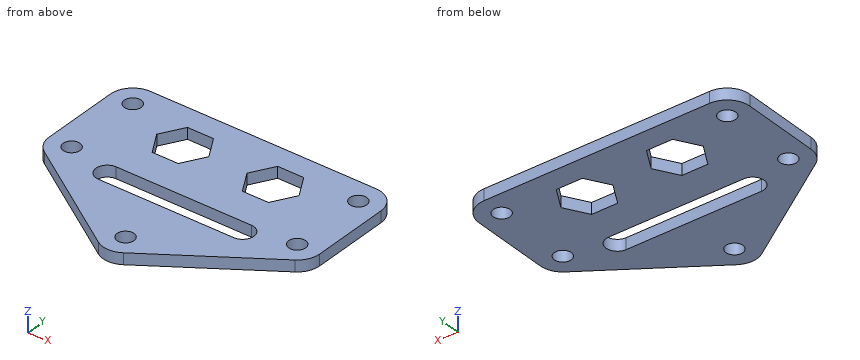
```python
from build123d import *

# Parameters (mm, degrees)
SKETCH1_R           = 4.7625
BOSS_EXTRUDE1_DEPTH = 6.35


with BuildPart() as part:
    # Sketch1 → Boss-Extrude1 (new body)
    with BuildSketch(Plane.XY):
        with BuildLine():
            Line((7.044692492, 4.696461661), (70.544692492, 47.029794995))
            ThreePointArc((70.544692492, 47.029794995), (74.697267404, 51.604238079), (76.2, 57.596833733))
            Line((76.2, 57.596833733), (76.2, 101.6))
            ThreePointArc((76.2, 101.6), (72.480256121, 110.580256121), (63.5, 114.3))
            Line((63.5, 114.3), (-63.5, 114.3))
            ThreePointArc((-63.5, 114.3), (-72.480256121, 110.580256121), (-76.2, 101.6))
            Line((-76.2, 101.6), (-76.2, 57.596833733))
            ThreePointArc((-76.2, 57.596833733), (-74.697267404, 51.604238079), (-70.544692492, 47.029794995))
            Line((-70.544692492, 47.029794995), (-7.044692492, 4.696461661))
            ThreePointArc((-7.044692492, 4.696461661), (0, 2.563500399), (7.044692492, 4.696461661))
        make_face()
        with Locations((-63.5, 101.6)):
            Circle(SKETCH1_R, mode=Mode.SUBTRACT)
        with Locations((-63.5, 57.596833733)):
            Circle(SKETCH1_R, mode=Mode.SUBTRACT)
        with Locations((63.5, 101.6)):
            Circle(SKETCH1_R, mode=Mode.SUBTRACT)
        with Locations((63.5, 57.596833733)):
            Circle(SKETCH1_R, mode=Mode.SUBTRACT)
        with Locations((0, 15.263500399)):
            Circle(SKETCH1_R, mode=Mode.SUBTRACT)
        with BuildLine():
            Line((-38.1, 57.15), (38.1, 57.15))
            ThreePointArc((38.1, 57.15), (44.45, 50.8), (38.1, 44.45))
            Line((38.1, 44.45), (-38.1, 44.45))
            ThreePointArc((-38.1, 44.45), (-44.45, 50.8), (-38.1, 57.15))
        make_face(mode=Mode.SUBTRACT)
        Polygon((-10.735303163, 88.9), (-18.067651581, 101.6), (-32.732348419, 101.6), (-40.064696837, 88.9), (-32.732348419, 76.2), (-18.067651581, 76.2), align=None, mode=Mode.SUBTRACT)
        Polygon((40.064696837, 88.9), (32.732348419, 101.6), (18.067651581, 101.6), (10.735303163, 88.9), (18.067651581, 76.2), (32.732348419, 76.2), align=None, mode=Mode.SUBTRACT)
    extrude(amount=BOSS_EXTRUDE1_DEPTH)


solid = part.part
```
Check sheet for the modelled part. Datum: model origin and axes. Units: mm. Coordinates: 2 decimals unless noted, no trailing zeros. Loops run counter-clockwise (first coordinate to the right, second up) from the corner with the lowest first, then second, coordinate; pieces in that order, holes last. Notation, with made-up numbers: M 63.5,60.5 L 90.5,60.5 A28 ccw 90.5,91.5 Z; hole C 6.25,53.25 d6. An arc over 180 degrees is marked long. Answer as a JSON object with one key per item and string values.
1. Scan lines: L1, parallel to X at y = 102, z = 1.75; L2, parallel to Y at x = 0, z = 3.5; L3, parallel to Y at x = 63.5, z = 3. Record each from-to range of solid material in increasing order. Write a range as from..to.
Outcome:
{"L1": "-76.19..-68.25, -58.75..58.75, 68.25..76.19", "L2": "2.56..10.5, 20.03..44.45, 57.15..114.3", "L3": "42.33..52.83, 62.36..96.84, 106.36..114.3"}
2. Sectioned sample at C-C on z = 2.25. Count the separate pieces of the cut face and the enclosed holes in it, and give its area (3 significant figures).
Outcome:
{"separate pieces": "1", "enclosed holes": "8", "area": "10,900 mm²"}
3. Sectioned sample at A-A on x = 0. Record the cut outline in (y, z), and give its area (3 significant figures).
Outcome:
{"outline": "M 2.56,0 L 10.5,0 L 10.5,6.35 L 2.56,6.35 Z; M 20.03,0 L 44.45,0 L 44.45,6.35 L 20.03,6.35 Z; M 57.15,0 L 114.3,0 L 114.3,6.35 L 57.15,6.35 Z", "area": "568 mm²"}
4. Depth check by flat-ended pin: P1, Ø1, axis at x = 42.5, y = 83, coming from the -Z side; P2, Ø3, axis at x = -28.5, z = 3, coming from the -Y side; P3, Ø5.5, axis at x = 0, y = 15.26, coming from the -Z side; P4, Ø1, axis at x = -51, z = 3, coming from the -Y side. Enter the tip coordinate at first touch or a pass-through.
Outcome:
{"P1": "z = 0", "P2": "y = 18", "P3": "through", "P4": "y = 33.67"}
5. Sectioned sample at B-B on y = 92.5. Record the cut outline in (x, z).
Outcome:
{"outline": "M -76.2,0 L -37.99,0 L -37.99,6.35 L -76.2,6.35 Z; M -12.81,0 L 12.81,0 L 12.81,6.35 L -12.81,6.35 Z; M 37.99,0 L 76.2,0 L 76.2,6.35 L 37.99,6.35 Z"}
